Input: dimensioned drawing with shaded views. Units: mm. Origin: part minimum x, y, z. A direction names the side the tool comes from. Round coordinates to 2 decimals unless told otherwise and drop trailing zeros. Loops run counter-clockwise (first coordinate to the right, second up) from the corner with the lowest first, then second, coordinate; pieces in that order, holes last. Notation, with made-up numbers: (40.5, -11) - (97.5, -11) arc R24 ccw to (97.5, 6) - close; hole circle Ø2 at (-28, -2.75). An arc over 180 degrees is marked (long way). One line per question, with ' | ' between items. Start each with the question number.
Item 1: Section B-B, the plane y = 21.5. Return loops of the section in (x, z), plus the area to 3 significant figures.
Item 2: Material intervals for line 1 along Z through (x, y) = (150, 19); line 2 along X through (y, z) = (17.25, 75); line 3 along Y through (x, z) = (196, 12), sorted ascending.
Item 3: Draft query along X for the marked faces 1, 2, 3 and 4. Return one class per face: pulls with the +X half, pulls with the -X half, needs draft (parallel to the pull), parting line crosses it, or undercut.
Item 4: First-contact query: pin 1 (2 mm diameter, centred on x = 78, y = 32.5, fed in from -Z); pin 2 (6 mm diameter, centred on x = 39.5, z = 21, fed in from +Y); pin 3 (1.5 mm diameter, centred on y = 32, z = 83.5, fed in from -X); pin 4 (12 mm diameter, centred on y = 38.5, z = 86.5, fed in from +X). Flat tips, straight axial feed; report the tip coordinate or a pass-through.
Item 5: Section C-C, the plane z = 100. Return loops of the section in (x, y).
Item 6: Section A-A, the plane x = 150. Return loops of the section in (y, z), plus the area to 3 significant figures.
Item 7: Section D-D, the plane y = 75.5. Return loops of the section in (x, z), plus the area to 3 significant figures.
Item 8: Set-up query: the marked faces 5 and 6. Return all of +Z, -Z, +X, -X, +Y, -Y with unobstructed straight access to the full face (end or side cutting, diameter ignored); none if empty.
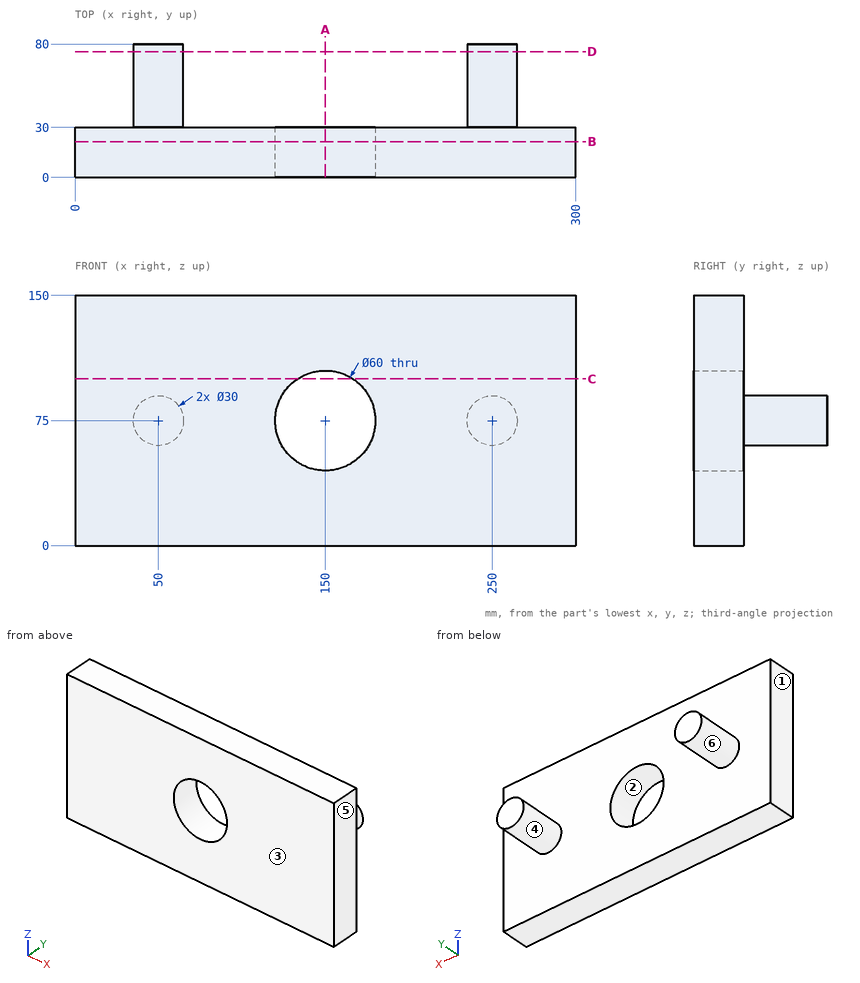
Return value:
1) outline: (0, 0) - (300, 0) - (300, 150) - (0, 150) - close; hole circle Ø60 at (150, 75) | area: 42,200 mm2
2) line 1: 0 to 45, 105 to 150 | line 2: 0 to 120, 180 to 300 | line 3: 0 to 30
3) face 1: pulls with the -X half | face 2: undercut | face 3: needs draft | face 4: undercut
4) pin 1: through | pin 2: y = 30 | pin 3: x = 37.16 | pin 4: x = 263.96
5) outline: (0, 0) - (133.42, 0) - (133.42, 30) - (0, 30) - close; (166.58, 0) - (300, 0) - (300, 30) - (166.58, 30) - close
6) outline: (0, 0) - (30, 0) - (30, 45) - (0, 45) - close; (0, 105) - (30, 105) - (30, 150) - (0, 150) - close | area: 2,700 mm2
7) outline: circle Ø30 at (50, 75); circle Ø30 at (250, 75) | area: 1,410 mm2
8) face 5: +Z, -Z, +X, +Y, -Y | face 6: +Y
